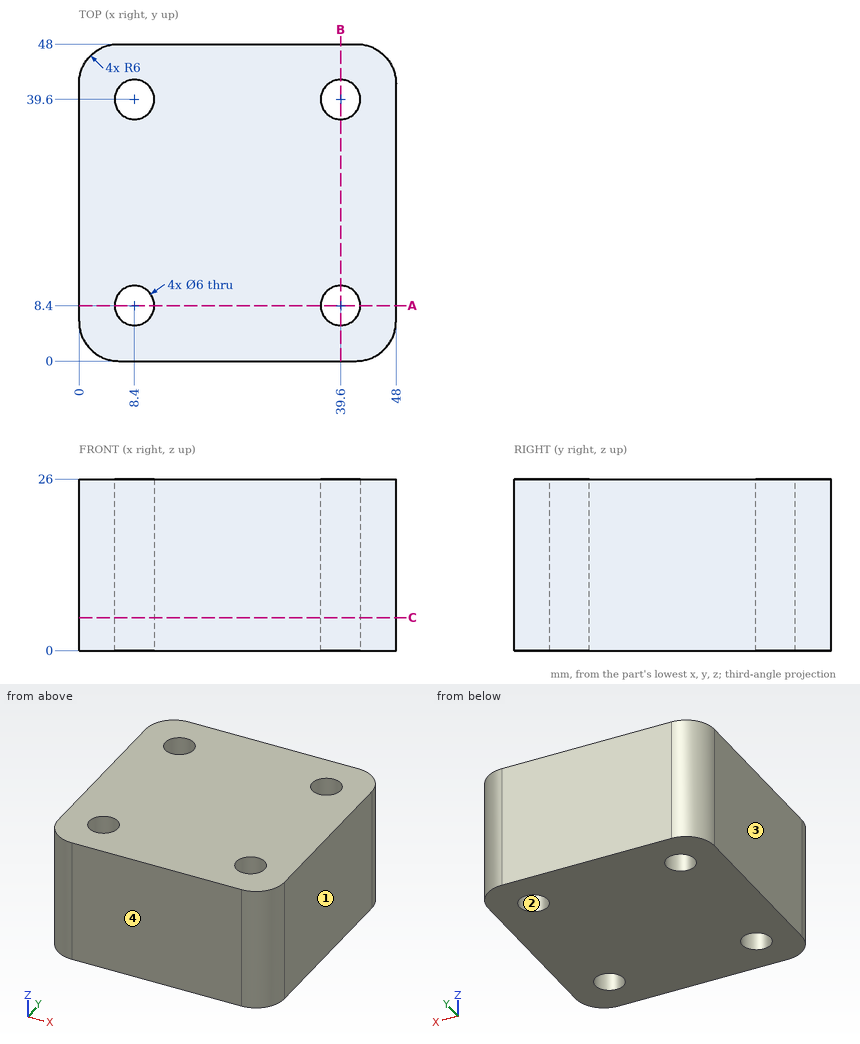
Geometry: see drawing. Coordinates: mm, zero at the bounding-box minimum. Round coordinates to 2 decimals unless told otherwise and drop trailing zeros. Write each loop counter-clockwise with the first axis right and the second up, starting at its lowest first coordinate (ties: lowest second). Pieces come first, ordered by that corner, then holes.
1) Draft query along X for the marked faces 1, 2, 3 and 4. Return one class per face: pulls with the +X half, pulls with the -X half, needs draft (parallel to the pull), parting line crosses it, or undercut.
2) Cut plane A-A (y = 8.4). Return the cut outline in (x, z).
3) Cut plane C-C (z = 5). Return the cut outline in (x, y).
4) Ray query, L1, parallel to Y at x = 8.4, z = 19.5; L2, parallel to X at y = 41.5, z = 19; L3, parallel to X at y = 9, z = 18. Return the intervals inside material, ascending.
Geometry says:
1. face 1: pulls with the +X half
1. face 2: undercut
1. face 3: pulls with the -X half
1. face 4: needs draft
2. outline: (0, 0) - (5.4, 0) - (5.4, 26) - (0, 26) - close; (11.4, 0) - (36.6, 0) - (36.6, 26) - (11.4, 26) - close; (42.6, 0) - (48, 0) - (48, 26) - (42.6, 26) - close
3. outline: (0, 6) arc R6 ccw to (6, 0) - (42, 0) arc R6 ccw to (48, 6) - (48, 42) arc R6 ccw to (42, 48) - (6, 48) arc R6 ccw to (0, 42) - close; hole circle Ø6 at (8.4, 8.4); hole circle Ø6 at (8.4, 39.6); hole circle Ø6 at (39.6, 8.4); hole circle Ø6 at (39.6, 39.6)
4. L1: y = 0 to 5.4, 11.4 to 36.6, 42.6 to 48
4. L2: x = 0 to 6.08, 10.72 to 37.28, 41.92 to 48
4. L3: x = 0 to 5.46, 11.34 to 36.66, 42.54 to 48
